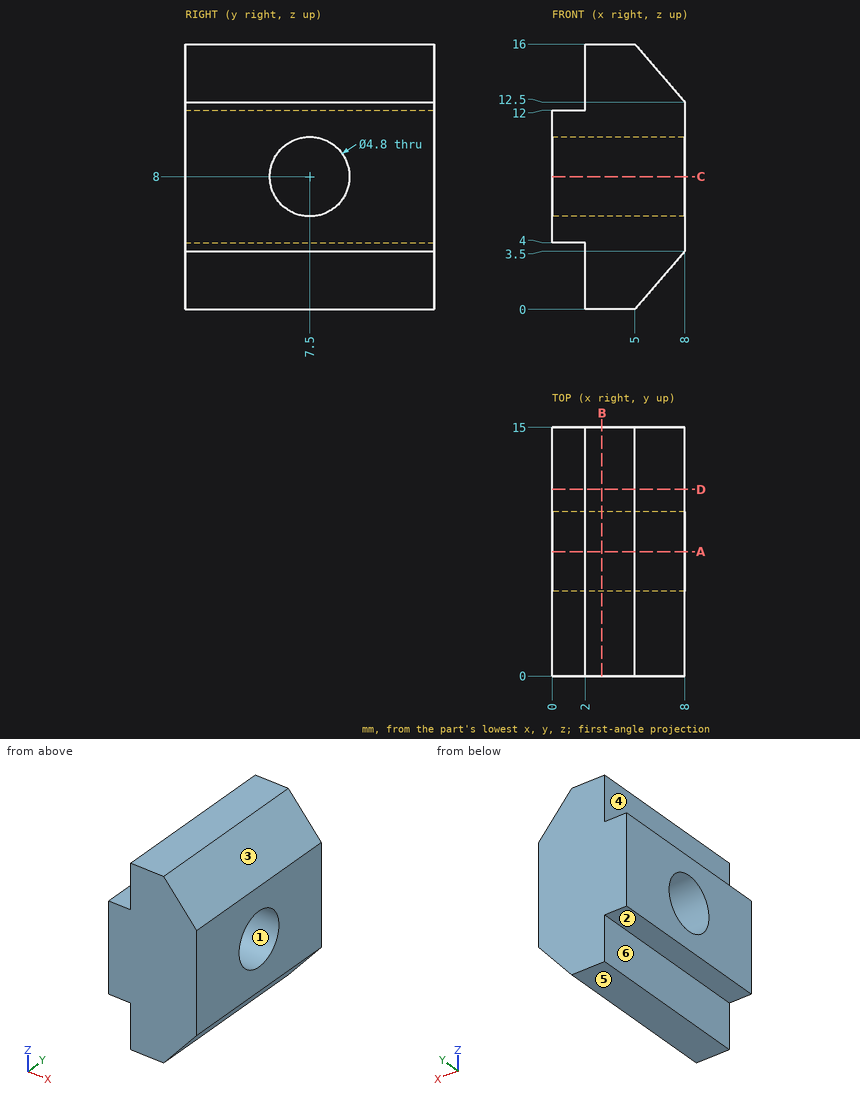
The drawing under review shows one solid part. Ordinate dimensions are in mm from its lowest x, y, z. A direction names the side the tool comes from. Round coordinates to 2 decimals unless told otherwise and drop trailing zeros. Write each loop counter-clockwise with the first axis right and the second up, starting at its lowest first coordinate (ties: lowest second). Pieces come first, ordered by that corner, then holes. Notation, with made-up numbers: M -1,48 L 3,48 A24 ccw 3,73 Z; hole C 28.25,-10 d5. An arc over 180 degrees is marked long. One line per item, written item: value. Start each with the question number.
(1) We need section D-D (y = 11.25). Give the boundary of the cut face in (x, z).
(2) Wall thickness on line 1 (Y direction, x = 6.25, z = 8); line 2 (Z direction, x = 4, y = 5.75); line 3 (Z direction, x = 4.25, y = 5.5): over which ranges is each line inside the solid? List them lowest first.
(3) Insertion check: pin 1 (1.2 mm diameter, centred on y = 11, z = 13, fed in from -X); pin 2 (4.5 mm diameter, centred on y = 7.5, z = 8, fed in from +X); pin 3 (0.6 mm diameter, centred on x = 1, y = 5.5, fed in from -Z); pin 4 (1.6 mm diameter, centred on x = 1, y = 9.5, fed in from +Z). Each pin has a flat end and moves straight along its axis. Give the tip position at first contact, or say it passes through.
(4) We need section C-C (z = 8). Give the boundary of the cut face in (x, y), and give its area (3 significant figures).
(5) The part is to be moulded in two halves that separate along Z. For the marked faces 1, 2 and 3, say which applies: released by +Z, released by -Z, zero draft, split by the parting line, or undercut.
(6) We need section A-A (y = 7.5). Give the boundary of the cut face in (x, z), and give its area (3 significant figures).
(7) We need section B-B (x = 3). Give the boundary of the cut face in (y, z), and give its area (3 significant figures).
(8) Machinability: for the marked faces 4, 5 and 6, which of the approach directions +Z, -Z, +X, -X, +Y, -Y give a long, thin tool a straight path to every point of the face, cutting with its end or side? Answer none if there is none.
Result:
1. outline: M 0,4 L 2,4 L 2,0 L 5,0 L 8,3.5 L 8,12.5 L 5,16 L 2,16 L 2,12 L 0,12 Z
2. line 1: 0 to 5.1, 9.9 to 15
2. line 2: 0 to 6.36, 9.64 to 16
2. line 3: 0 to 6.67, 9.33 to 16
3. pin 1: x = 2
3. pin 2: through
3. pin 3: z = 4
3. pin 4: z = 12
4. outline: M 0,0 L 8,0 L 8,5.1 L 0,5.1 Z; M 0,9.9 L 8,9.9 L 8,15 L 0,15 Z
4. area: 81.6 mm²
5. face 1: undercut
5. face 2: released by -Z
5. face 3: released by +Z
6. outline: M 0,4 L 2,4 L 2,0 L 5,0 L 8,3.5 L 8,5.6 L 0,5.6 Z; M 0,10.4 L 8,10.4 L 8,12.5 L 5,16 L 2,16 L 2,12 L 0,12 Z
6. area: 63.1 mm²
7. outline: M 0,0 L 15,0 L 15,16 L 0,16 Z; hole C 7.5,8 d4.8
7. area: 222 mm²
8. face 4: +Z, -X, +Y, -Y
8. face 5: -Z, +X, -X, +Y, -Y
8. face 6: -Z, -X, +Y, -Y
